from build123d import *

# Parameters (mm, degrees)
SKICA1_W             = 18
SKICA1_H             = 19.2
BODY_SMALL_DEPTH     = 0.8
SKICA2_W             = 18
SKICA2_H             = 6.3
BODY_EXTENSION_DEPTH = 0.8
SKICA3_R             = 0.284
VIAS_DEPTH           = 19.287974191
ANTENNA_DEPTH        = 0.018


with BuildPart() as part:
    # Skica1 → body_small (new body)
    with BuildSketch(Plane.XY):
        Rectangle(SKICA1_W, SKICA1_H)
    extrude(amount=BODY_SMALL_DEPTH)

    # Skica2 → body_extension (add)
    with BuildSketch(Plane(origin=(0, 0, 0), x_dir=(-1, 0, 0), z_dir=(0, 0, -1))):
        with Locations((0, 12.75)):
            Rectangle(SKICA2_W, SKICA2_H)
    extrude(amount=-BODY_EXTENSION_DEPTH)

    # Skica3 → vias (cut, through all)
    with BuildSketch(Plane.XY.offset(0.8)):
        with Locations((-6.985, -9.6)):
            Circle(SKICA3_R)
        with Locations((-9, -8.1)):
            Circle(SKICA3_R)
        with Locations((9, -8.1)):
            Circle(SKICA3_R)
        with Locations((-9, -6.83)):
            Circle(SKICA3_R)
        with Locations((9, -6.83)):
            Circle(SKICA3_R)
        with Locations((-9, -5.56)):
            Circle(SKICA3_R)
        with Locations((9, -5.56)):
            Circle(SKICA3_R)
        with Locations((-9, -4.29)):
            Circle(SKICA3_R)
        with Locations((9, -4.29)):
            Circle(SKICA3_R)
        with Locations((-9, -3.02)):
            Circle(SKICA3_R)
        with Locations((9, -3.02)):
            Circle(SKICA3_R)
        with Locations((-9, -1.75)):
            Circle(SKICA3_R)
        with Locations((9, -1.75)):
            Circle(SKICA3_R)
        with Locations((-9, -0.48)):
            Circle(SKICA3_R)
        with Locations((9, -0.48)):
            Circle(SKICA3_R)
        with Locations((-9, 0.79)):
            Circle(SKICA3_R)
        with Locations((9, 0.79)):
            Circle(SKICA3_R)
        with Locations((-9, 2.06)):
            Circle(SKICA3_R)
        with Locations((9, 2.06)):
            Circle(SKICA3_R)
        with Locations((-9, 3.33)):
            Circle(SKICA3_R)
        with Locations((9, 3.33)):
            Circle(SKICA3_R)
        with Locations((-9, 4.6)):
            Circle(SKICA3_R)
        with Locations((9, 4.6)):
            Circle(SKICA3_R)
        with Locations((-9, 5.87)):
            Circle(SKICA3_R)
        with Locations((9, 5.87)):
            Circle(SKICA3_R)
        with Locations((-9, 7.14)):
            Circle(SKICA3_R)
        with Locations((9, 7.14)):
            Circle(SKICA3_R)
        with Locations((-9, 8.41)):
            Circle(SKICA3_R)
        with Locations((9, 8.41)):
            Circle(SKICA3_R)
        with Locations((-5.715, -9.6)):
            Circle(SKICA3_R)
        with Locations((-4.445, -9.6)):
            Circle(SKICA3_R)
        with Locations((-3.175, -9.6)):
            Circle(SKICA3_R)
        with Locations((-1.905, -9.6)):
            Circle(SKICA3_R)
        with Locations((-0.635, -9.6)):
            Circle(SKICA3_R)
        with Locations((0.635, -9.6)):
            Circle(SKICA3_R)
        with Locations((1.905, -9.6)):
            Circle(SKICA3_R)
        with Locations((3.175, -9.6)):
            Circle(SKICA3_R)
        with Locations((4.445, -9.6)):
            Circle(SKICA3_R)
        with Locations((5.715, -9.6)):
            Circle(SKICA3_R)
        with Locations((6.985, -9.6)):
            Circle(SKICA3_R)
    extrude(amount=-VIAS_DEPTH, mode=Mode.SUBTRACT)

    # Skica4 → antenna (add)
    with BuildSketch(Plane.XY.offset(0.8)):
        Polygon((-7, 11.8), (-6, 11.8), (-6, 14.3), (-5, 14.3), (-5, 12.4), (-1.75, 12.4), (-1.75, 14.3), (-0.75, 14.3), (-0.75, 12.4), (2.5, 12.4), (2.5, 14.3), (3.5, 14.3), (3.5, 7.68), (4.5, 7.68), (4.5, 14.3), (5.5, 14.3), (5.5, 7.68), (6.5, 7.68), (6.5, 15.3), (1.5, 15.3), (1.5, 13.4), (0.25, 13.4), (0.25, 15.3), (-2.75, 15.3), (-2.75, 13.4), (-4, 13.4), (-4, 15.3), (-7, 15.3), align=None)
    extrude(amount=ANTENNA_DEPTH)


solid = part.part
Build history of the part. All positions in model axes, mm. Coordinates: 2 decimals unless noted, no trailing zeros. Order: outer loops, then holes, each group sorted by start corner. A loop starts at its lowest first (then second) coordinate and runs counter-clockwise, first axis right, second up. Notation, with made-up numbers: (89.5, -21) - (148.5, -21) arc R29 ccw to (148.5, 6) - close; hole circle Ø2 at (-31.5, -34). An arc over 180 degrees is marked (long way). Write each question's results on one line, items separated by ' | '. Start each with the question number.
Item 1: Flat gauge pin, fed straight in: pin 1 (10 mm diameter, centred on x = 0, y = -2.5, fed in from +Z). Where does the tip first touch, or does it go through?
Item 2: Wall check: probe 1 along Z at (x, y) = (-4.5, 11.25); probe 2 along Y at (x, z) = (7, 0.5); probe 3 along X at (y, z) = (-1.75, 0.15). Give the ranges that are in metal, low to high. Write a range as [from, to].
Item 3: Band-saw the part on D-D on y = -1.75. Write the cut outline in (x, z), and give its area (3 significant figures).
Numbers:
1) pin 1: z = 0.8
2) probe 1: [0, 0.8] | probe 2: [-9.32, 15.9] | probe 3: [-8.72, 8.72]
3) outline: (-8.72, 0) - (8.72, 0) - (8.72, 0.8) - (-8.72, 0.8) - close | area: 13.9 mm^2
